from build123d import *

# Parameters (mm, degrees)
F0_W     = 100
F0_H     = 68
F1_DEPTH = 6
F2_D     = 3.3
F3_D     = 4


with BuildPart() as f1:
    # F0 (on Top) → F1 (new body)
    with BuildSketch(Plane.XY):
        with Locations((-7.0588196459, -1.6911783814)):
            Rectangle(F0_W, F0_H)
    extrude(amount=-F1_DEPTH)

    # F2 (through all)
    with Locations(Plane.XY):
        with Locations((-51.0588196459, 20.8088216186), (-23.0588196459, 20.8088216186), (-51.0588196459, -24.1911783814), (-23.0588196459, -24.1911783814), (8.9411803541, 20.8088216186), (36.9411803541, 20.8088216186), (8.9411803541, -24.1911783814), (36.9411803541, -24.1911783814)):
            Hole(F2_D / 2)

    # F3 (through all)
    with Locations(Plane.XY):
        with Locations((-14.0588196459, -17.6911783814), (-0.0588196459, -17.6911783814)):
            Hole(F3_D / 2)


solid = f1.part
The model under review builds one solid part; all positions refer to its coordinate system, in mm. Round coordinates to 2 decimals unless told otherwise and drop trailing zeros. Order: outer loops, then holes, each group sorted by start corner. A loop starts at its lowest first (then second) coordinate and runs counter-clockwise, first axis right, second up. Notation, with made-up numbers: (14, 1.25) -> (49, 1.25) arc R26 cw to (49, 26.25) -> close; hole circle Ø5 at (55, 45). An arc over 180 degrees is marked (long way). Write item = value, one per line. Start each with the question number.
Item 1: Mouldability with a two-part tool opening along Y and no side actions: class faces 1 (the face through (-8, 32.309, -3)), 2 (the face through (42.941, -2, -3)), 3 (the face through (-8, -35.691, -3)), 4 (the face through (7.367, -23.696, -3.042)) as released by +Y, released by -Y, zero draft, split by the parting line, or undercut.
Item 2: Consider section A-A on x = -0.5. Write out the cut boundary in (y, z), plus the area to 3 significant figures.
Item 3: For line 1 along Y through (x, z) = (-51.5, -3.25); line 2 along Y through (x, z) = (35.5, -2.2), list the stretches that pass through material, from the lowest coordinate up.
Item 4: Clearance check with a flat-ended pin moving along its axis: pin 1 Ø3 at (x, y) = (-23.06, 20.81) entering from -Z. State where the tip first meets the part, or that it passes through.
Conclusion:
q1.face_1 = released by +Y
q1.face_2 = zero draft
q1.face_3 = released by -Y
q1.face_4 = undercut
q2.outline = (-35.69, -6) -> (-19.64, -6) -> (-19.64, 0) -> (-35.69, 0) -> close; (-15.74, -6) -> (32.31, -6) -> (32.31, 0) -> (-15.74, 0) -> close
q2.area = 385 mm2
q3.line_1 = -35.69 to -25.78, -22.6 to 19.22, 22.4 to 32.31
q3.line_2 = -35.69 to -24.99, -23.39 to 20.01, 21.61 to 32.31
q4.pin_1 = through
